Part print with two shaded views. Sizes in mm from the minimum x, y, z corner. Coordinates: 2 decimals unless noted, no trailing zeros. Order: outer loops, then holes, each group sorted by start corner. A loop starts at its lowest first (then second) coordinate and runs counter-clockwise, first axis right, second up. Notation, with made-up numbers: (67.5, 64.5) - (119.5, 64.5) arc R37 cw to (119.5, 100.5) - close; hole circle Ø2 at (36, 85). An arc over 180 degrees is marked (long way). Return JSON: item names as keys, results as strings.
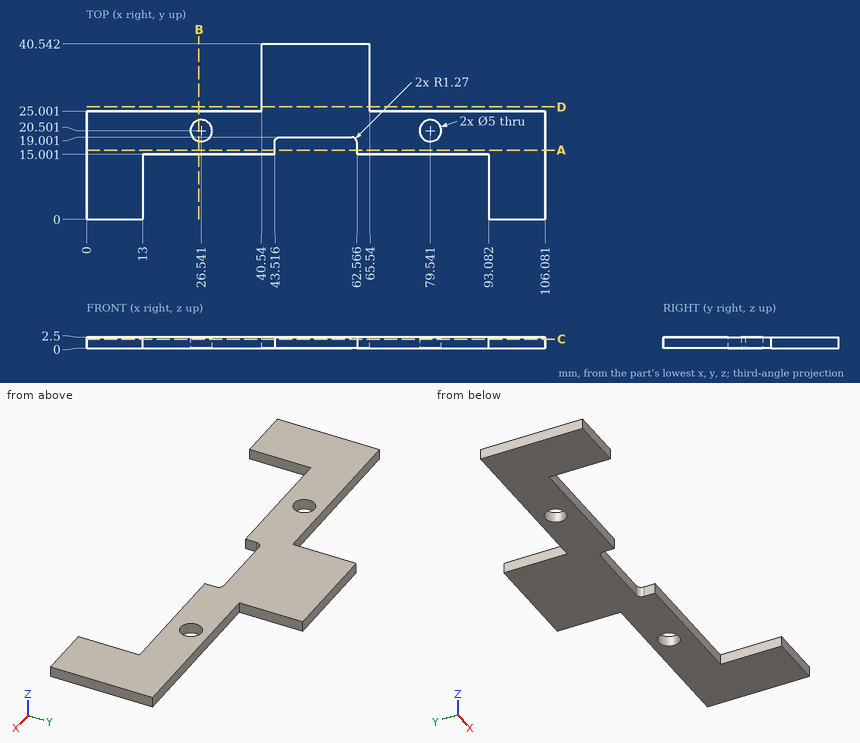
Item 1: Wall check: L1, parallel to X at y = 20.5, z = 2.4; L2, parallel to X at y = 15.5, z = 1.35; L3, parallel to Y at x = 70.5, z = 0.95. Give the ranges that are in metal, low to high. Write a range as [from, to].
Findings below:
{"L1": "x = [0, 24.04], [29.04, 77.04], [82.04, 106.08]", "L2": "x = [0, 43.52], [62.57, 106.08]", "L3": "y = [15, 25]"}
Item 2: Band-saw the part on C-C, the plane z = 2.1. List the corners of the cut face in (x, y).
Findings below:
{"outline": "(0, 0) - (13, 0) - (13, 15) - (43.52, 15) - (43.52, 17.73) arc R1.27 cw to (44.79, 19) - (61.3, 19) arc R1.27 cw to (62.57, 17.73) - (62.57, 15) - (93.08, 15) - (93.08, 0) - (106.08, 0) - (106.08, 25) - (65.54, 25) - (65.54, 40.54) - (40.54, 40.54) - (40.54, 25) - (0, 25) - close; hole circle Ø5 at (26.54, 20.5); hole circle Ø5 at (79.54, 20.5)"}
Item 3: Band-saw the part on D-D, the plane y = 26. List the corners of the cut face in (x, z).
Findings below:
{"outline": "(40.54, 0) - (65.54, 0) - (65.54, 2.5) - (40.54, 2.5) - close"}
Item 4: Band-saw the part on B-B, the plane x = 26. List the corners of the cut face in (y, z).
Findings below:
{"outline": "(15, 0) - (18.06, 0) - (18.06, 2.5) - (15, 2.5) - close; (22.94, 0) - (25, 0) - (25, 2.5) - (22.94, 2.5) - close"}
Item 5: Band-saw the part on A-A, the plane y = 16. List the corners of the cut face in (x, z).
Findings below:
{"outline": "(0, 0) - (43.52, 0) - (43.52, 2.5) - (0, 2.5) - close; (62.57, 0) - (106.08, 0) - (106.08, 2.5) - (62.57, 2.5) - close"}
Item 6: Drop flat-ended pins along their axis: P1, Ø0.8, axis at x = 17, z = 0.5, coming from the +Y side; P2, Ø1.2, axis at x = 29.5, z = 1, coming from the -Y side; P3, Ø12, axis at x = 66.5, y = 12, coming from the -Z side. Give the stop position or say it passes through.
Findings below:
{"P1": "stops at y = 25", "P2": "stops at y = 15", "P3": "stops at z = 0"}
